Source: three-view drawing plus pictorial views. Frame: mm from the lowest corner of the part. A direction names the side the tool comes from. Give positions to 0.01 mm unless a question says otherwise; leave off trailing zeros. Loops run counter-clockwise (first coordinate to the right, second up) from the corner with the lowest first, then second, coordinate; pieces in that order, holes last. Notation, with made-up numbers: (56.25, 7.25) -> (83.25, 7.25) arc R26 cw to (83.25, 24.25) -> close; hole circle Ø7 at (-4, 31). An arc over 180 degrees is marked (long way). Answer in a Markdown table with one row per item. Add a question column.
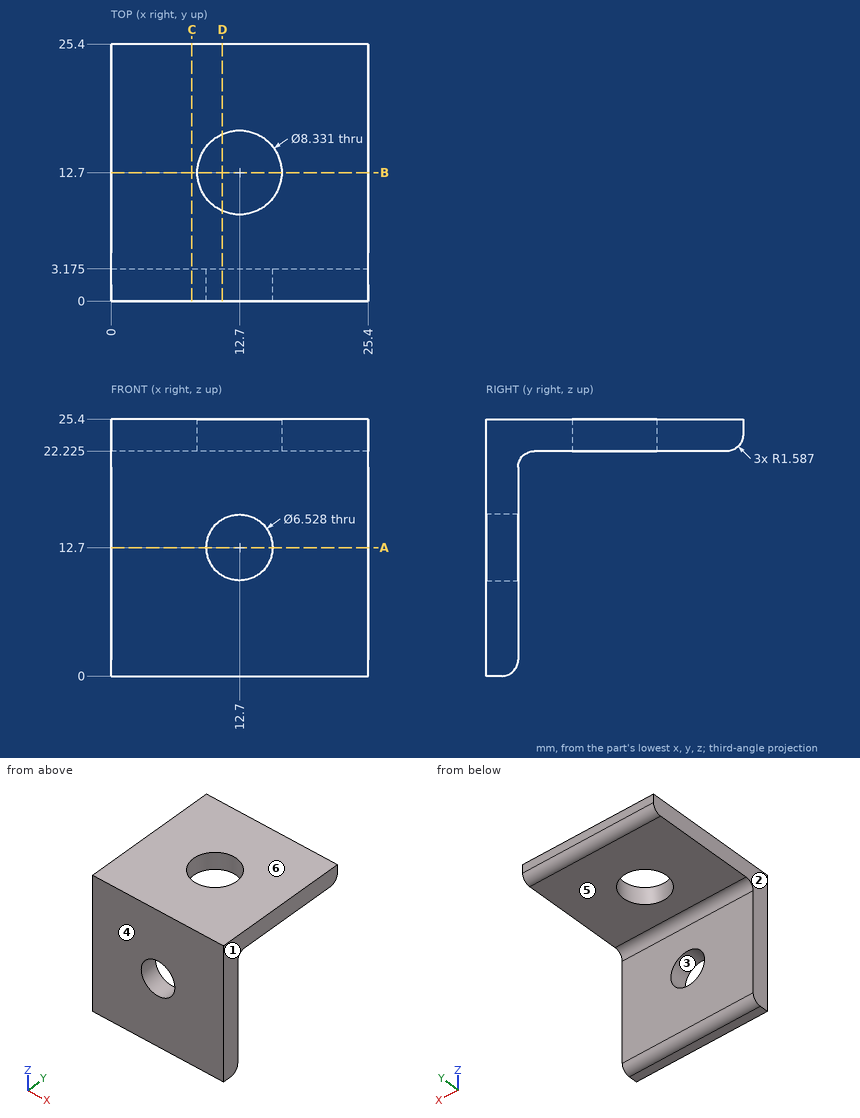
(1) Cut plane A-A on z = 12.7. Return the cut outline in (x, y) (1 decimal).
(2) Pin query (flat end, axial travel): pin 1 Ø8 at (x, z) = (20, 11.5) entering from +Y (1 decimal); pin 2 Ø15 at (x, y) = (14.5, 13.5) entering from -Z (1 decimal). Return the tip coordinate at first contact, or that it passes through.
(3) Cut plane B-B on y = 12.7. Return the cut outline in (x, z) (1 decimal).
(4) Cut plane D-D on x = 11. Return the cut outline in (y, z) (1 decimal), then the cut area to 3 significant figures.
(5) Cut plane C-C on x = 8. Return the cut outline in (y, z) (1 decimal).
(6) Material intervals for line 1 along X through (y, z) = (2.15, 12.7); line 2 along Y through (x, z) = (12.7, 24.2) (1 decimal); line 3 along Y through (x, z) = (18.75, 15.75) (1 decimal), sorted ascending. Write a range as from..to.
(7) Reachability of the marked faces 5 and 6 from +Z, -Z, +X, -X, +Y, -Y: full face, straight path, thin tool, end or side. Return the list, or none.
(8) Draft query along X for the marked faces 1, 2, 3 and 4. Return one class per face: +X half, -X half, draft (parallel to the pull), parting line (faces both ways), or undercut.
Answer list:
| question | item | result |
|---|---|---|
| 1 | outline | (0, 0) -> (9.4, 0) -> (9.4, 3.2) -> (0, 3.2) -> close; (16, 0) -> (25.4, 0) -> (25.4, 3.2) -> (16, 3.2) -> close |
| 2 | pin 1 | stops at y = 3.2 |
| 2 | pin 2 | stops at z = 22.2 |
| 3 | outline | (0, 22.2) -> (8.5, 22.2) -> (8.5, 25.4) -> (0, 25.4) -> close; (16.9, 22.2) -> (25.4, 22.2) -> (25.4, 25.4) -> (16.9, 25.4) -> close |
| 4 | outline | (0, 0) -> (1.6, 0) arc R1.6 ccw to (3.2, 1.6) -> (3.2, 9.9) -> (0, 9.9) -> close; (0, 15.5) -> (3.2, 15.5) -> (3.2, 20.6) arc R1.6 cw to (4.8, 22.2) -> (8.9, 22.2) -> (8.9, 25.4) -> (0, 25.4) -> close; (16.5, 22.2) -> (23.8, 22.2) arc R1.6 ccw to (25.4, 23.8) -> (25.4, 25.4) -> (16.5, 25.4) -> close |
| 4 | area | 109 mm² |
| 5 | outline | (0, 0) -> (1.6, 0) arc R1.6 ccw to (3.2, 1.6) -> (3.2, 20.6) arc R1.6 cw to (4.8, 22.2) -> (23.8, 22.2) arc R1.6 ccw to (25.4, 23.8) -> (25.4, 25.4) -> (0, 25.4) -> close |
| 6 | line 1 | x = 0..9.44, 15.96..25.4 |
| 6 | line 2 | y = 0..8.5, 16.9..25.4 |
| 6 | line 3 | y = 0..3.2 |
| 7 | face 5 | -Z, +X, -X, +Y |
| 7 | face 6 | +Z, +X, -X, +Y, -Y |
| 8 | face 1 | +X half |
| 8 | face 2 | -X half |
| 8 | face 3 | undercut |
| 8 | face 4 | draft |
